Could you check a few things on this model? Use its own coordinates, in mm. A direction names the side the tool comes from. Round coordinates to 2 decimals unless told otherwise and drop trailing zeros. Write each loop counter-clockwise with the first axis right and the second up, starting at its lowest first coordinate (ties: lowest second). Pieces come first, ordered by that corner, then holes. Notation, with made-up numbers: (-6, 23.5) -> (11, 23.5) arc R10 cw to (11, 34.5) -> close; hole circle Ø3 at (27, 21.25). An arc over 180 degrees is marked (long way). Answer as CSV lines item,"result". Start each with the question number.
Q1. If we mould it in two halves opening along Z, with no side actions, what happens to faces 3 (the cylindrical face through (6.439, 55.376, 12.052)), 4 (the flat face through (6, -1, 41.275)), 5 (the flat face through (6, 76.2, 1))? For each: pulls with the +Z half, pulls with the -Z half, needs draft (parallel to the pull), parting line crosses it, or undercut.
Q2. Imagine slicing it at C-C on x = 10.5. Please give me the cut outline in (y, z) (3 decimals), and give its area (3 significant figures).
Q3. For faces 1 (the flat face through (6, -76.2, 1)), 2 (the cylindrical face through (0.493, 0.33, -17.018)), which set-ups out of +Z, -Z, +X, -X, +Y, -Y let a thin tool reach every point of the face, with its end or its side?
Q4. Imagine slicing it at A-A on y = 57.15. Please give me the cut outline in (x, z) (3 decimals).
Q5. Imagine slicing it at B-B on y = 0. Please give me the cut outline in (x, z) (3 decimals), and give its area (3 significant figures).
Q6. If I drill on line 1 (Y direction, x = 10, z = 12); line 2 (Y direction, x = 8, z = -9); line 3 (Y direction, x = 8.25, z = -6.5), over which ranges is the centre line in solid material (lowest first)? Write a range as [from, to].
from build123d import *

# Parameters (mm, degrees)
ESQUISSE1_W             = 82.55
ESQUISSE1_H             = 152.4
BOSS_EXTRU_1_DEPTH      = 12.7
ESQUISSE2_R             = 2
ENL_V_MAT_EXTRU_1_DEPTH = 88.586275323
ESQUISSE3_R             = 7
ENL_V_MAT_EXTRU_2_DEPTH = 88.586275323
ESQUISSE5_R             = 7.5
ENL_V_MAT_EXTRU_4_DEPTH = 1


with BuildPart() as part:
    # Esquisse1 → Boss.-Extru.1 (new body)
    with BuildSketch(Plane(origin=(0, 0, 0), x_dir=(0, 0, -1), z_dir=(1, 0, 0))):
        Rectangle(ESQUISSE1_W, ESQUISSE1_H)
    extrude(amount=BOSS_EXTRU_1_DEPTH)

    # Esquisse2 → Enlèv. mat.-Extru.1 (cut, through all)
    with BuildSketch(Plane(origin=(12.7, 0, 0), x_dir=(0, 0, -1), z_dir=(1, 0, 0))):
        with Locations((-12.974999958, 57.15)):
            Circle(ESQUISSE2_R)
        with Locations((32.025000042, 57.15)):
            Circle(ESQUISSE2_R)
        with Locations((-12.974999958, -57.15)):
            Circle(ESQUISSE2_R)
        with Locations((32.025000042, -57.15)):
            Circle(ESQUISSE2_R)
    extrude(amount=-ENL_V_MAT_EXTRU_1_DEPTH, mode=Mode.SUBTRACT)

    # Esquisse3 → Enlèv. mat.-Extru.2 (cut, through all)
    with BuildSketch(Plane(origin=(12.7, 0, 0), x_dir=(0, 0, -1), z_dir=(1, 0, 0))):
        with Locations((9.525, 0)):
            Circle(ESQUISSE3_R)
    extrude(amount=-ENL_V_MAT_EXTRU_2_DEPTH, mode=Mode.SUBTRACT)

    # Esquisse5 → Enlèv. mat.-Extru.4 (cut)
    with BuildSketch(Plane.ZY):
        with Locations((-9.525, 0)):
            Circle(ESQUISSE5_R)
    extrude(amount=-ENL_V_MAT_EXTRU_4_DEPTH, mode=Mode.SUBTRACT)


solid = part.part
Checks:
1,face 3,"undercut"
1,face 4,"pulls with the +Z half"
1,face 5,"needs draft"
2,outline,"(-76.2, -41.275) -> (76.2, -41.275) -> (76.2, 41.275) -> (-76.2, 41.275) -> close; hole circle Ø4 at (-57.15, -32.025); hole circle Ø4 at (-57.15, 12.975); hole circle Ø14 at (0, -9.525); hole circle Ø4 at (57.15, -32.025); hole circle Ø4 at (57.15, 12.975)"
2,area,"12,400 mm^2"
3,face 1,"+Z, -Z, +X, -X, -Y"
3,face 2,"-X"
4,outline,"(0, -41.275) -> (12.7, -41.275) -> (12.7, -34.025) -> (0, -34.025) -> close; (0, -30.025) -> (12.7, -30.025) -> (12.7, 10.975) -> (0, 10.975) -> close; (0, 14.975) -> (12.7, 14.975) -> (12.7, 41.275) -> (0, 41.275) -> close"
5,outline,"(0, -41.275) -> (12.7, -41.275) -> (12.7, -16.525) -> (1, -16.525) -> (1, -17.025) -> (0, -17.025) -> close; (0, -2.025) -> (1, -2.025) -> (1, -2.525) -> (12.7, -2.525) -> (12.7, 41.275) -> (0, 41.275) -> close"
5,area,"870 mm^2"
6,line 1,"[-76.2, -58.9], [-55.4, 55.4], [58.9, 76.2]"
6,line 2,"[-76.2, -6.98], [6.98, 76.2]"
6,line 3,"[-76.2, -6.31], [6.31, 76.2]"
